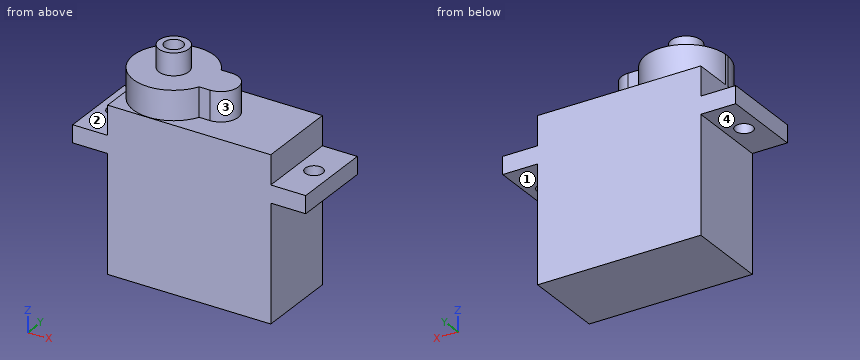
```python
from build123d import *

# Parameters (mm, degrees)
P_IDAT_VYSUNUT_M1_DEPTH  = 5.555
P_IDAT_VYSUNUT_M2_DEPTH  = 4
SKICA3_R                 = 2.03883748
SKICA3_R_2               = 1.24519559
P_IDAT_VYSUNUT_M3_DEPTH  = 3
SKICA5_R                 = 1.190602913
SKICA5_R_2               = 1.19060243
ODEBRAT_VYSUNUT_M1_DEPTH = 23


# Read off the part's stored shape, not the designer's step: Přidat vysunutím2
with BuildPart() as part:
    # Skica1 → Přidat vysunutím1 (new, symmetric)
    with BuildSketch(Plane(origin=(0, 0, 0), x_dir=(1, 0, 0), z_dir=(0, 1, 0))):
        Polygon((11.32935, -15.875), (16.09185, -15.875), (16.09185, -18.25625), (11.32935, -18.25625), (11.32935, -22.225), (-10.89565, -22.225), (-10.89565, -18.25625), (-15.65815, -18.25625), (-15.65815, -15.875), (-10.89565, -15.875), (-10.89565, 0), (11.32935, 0), align=None)
    extrude(amount=P_IDAT_VYSUNUT_M1_DEPTH, both=True)

    # Přidat vysunutím2 outline → Přidat vysunutím2 (add)
    with BuildSketch(Plane.XY.offset(22.225)):
        with BuildLine():
            Line((-10.89565, 0.263816958), (-10.89565, -0.263816958))
            ThreePointArc((-10.89565, -0.263816958), (-6.494080203, -5.390484118), (-0.444197365, -2.381256561))
            Line((-0.444197365, -2.381256561), (1.010536018, -2.381256561))
            ThreePointArc((1.010536018, -2.381256561), (3.391829299, 2.729e-06), (1.010604, 2.38133))
            Line((1.010604, 2.38133), (-0.444232639, 2.38133))
            ThreePointArc((-0.444232639, 2.38133), (-6.494120128, 5.390476029), (-10.89565, 0.263816958))
        make_face()
    extrude(amount=P_IDAT_VYSUNUT_M2_DEPTH)

    # Skica3 → Přidat vysunutím3 (add)
    with BuildSketch(Plane.XY.offset(26.225)):
        with Locations((-5.401980861, 0)):
            Circle(SKICA3_R)
        with Locations((-5.401980861, 0)):
            Circle(SKICA3_R_2, mode=Mode.SUBTRACT)
    extrude(amount=P_IDAT_VYSUNUT_M3_DEPTH)

    # Skica5 → Odebrat vysunutím1 (cut)
    with BuildSketch(Plane.XY.offset(18.25625)):
        with Locations((-13.276937552, 5.8558e-05)):
            Circle(SKICA5_R)
        with Locations((13.71053658, 6.1415e-05)):
            Circle(SKICA5_R_2)
    extrude(amount=-ODEBRAT_VYSUNUT_M1_DEPTH, mode=Mode.SUBTRACT)


solid = part.part
```
Can you work these out from the model? Positions are in its coordinate system, mm. Face numbers are marked on the shaded views. A direction names the side the tool comes from. Give positions to 0.01 mm unless a question says otherwise; leave off trailing zeros. Write each loop counter-clockwise with the first axis right and the second up, starting at its lowest first coordinate (ties: lowest second). Pieces come first, ordered by that corner, then holes. Notation, with made-up numbers: (-36.75, 45.5) - (-18.75, 45.5) arc R22 ccw to (-18.75, 58.5) - close; hole circle Ø10 at (3.5, 8). An arc over 180 degrees is marked (long way). Write item = value, one per line. Start each with the question number.
1. Imagine slicing it at A-A (y = 0.75). Count the separate pieces of the cut face and the enclosed holes in it, and give its area (3 significant figures).
2. Please list where these lines run through material, in increasing order: line 1 (Z direction, x = 13, y = -4) (3 decimals); line 2 (X direction, y = -0.25, z = 16.5); line 3 (Z direction, x = -10, y = -0.25) (3 decimals).
3. For pin 1 (0.7 mm diameter, centred on x = -5, y = 0, fed in from +Z) (3 decimals); pin 2 (5 mm diameter, centred on y = 2.5, z = 25, fed in from +X); pin 3 (3.5 mm diameter, centred on y = -2, z = 9.5, fed in from +X), each with a flat end and sliding along its axis, tell me the tip position at first contact or that it passes through.
4. Imagine slicing it at C-C (y = 4.75). Please give me the cut outline in (x, z) (3 decimals), and give its area (3 significant figures).
5. Imagine slicing it at D-D (x = 5.5). Please give me the cut outline in (y, z) (3 decimals), and give its area (3 significant figures).
6. On a 3-axis mill with a long thin cutter (end or side, diameter ignored), from which of +Z, -Z, +X, -X, +Y, -Y can I reach the whole of each face in a straight line? I mean the marked faces 1, 2, 3 and 4. Say none if no direction works.
7. Imagine slicing it at B-B (z = 24). Please give me the cut outline in (x, y).
Worked answers:
q1.separate_pieces = 3
q1.enclosed_holes = 0
q1.area = 570 mm2
q2.line_1 = 15.875 to 18.256
q2.line_2 = -15.66 to -14.44, -12.11 to 12.55, 14.87 to 16.09
q2.line_3 = 0 to 26.225
q3.pin_1 = 26.225
q3.pin_2 = 3.39
q3.pin_3 = 11.33
q4.outline = (-15.658, 15.875) - (-10.896, 15.875) - (-10.896, 0) - (11.329, 0) - (11.329, 15.875) - (16.092, 15.875) - (16.092, 18.256) - (11.329, 18.256) - (11.329, 22.225) - (-2.629, 22.225) - (-2.629, 26.225) - (-8.175, 26.225) - (-8.175, 22.225) - (-10.896, 22.225) - (-10.896, 18.256) - (-15.658, 18.256) - close
q4.area = 539 mm2
q5.outline = (-5.555, 0) - (5.555, 0) - (5.555, 22.225) - (-5.555, 22.225) - close
q5.area = 247 mm2
q6.face_1 = -Z, +X, +Y, -Y
q6.face_2 = +Z, -X, +Y, -Y
q6.face_3 = +Z, +X
q6.face_4 = -Z, -X, +Y, -Y
q7.outline = (-10.9, -0.26) arc R5.5 ccw to (-0.44, -2.38) - (1.01, -2.38) arc R2.38 ccw to (1.01, 2.38) - (-0.44, 2.38) arc R5.5 ccw to (-10.9, 0.26) - close
